Part model, mm, in its own coordinate system. A direction names the side the tool comes from. Give positions to 0.01 mm unless a question says otherwise; leave off trailing zeros. Write each loop counter-clockwise with the first axis right and the second up, starting at its lowest first coordinate (ties: lowest second). Pieces come first, ordered by that corner, then holes. Notation, with made-up numbers: M 84.5,29 L 110.5,29 A28 ccw 110.5,54 Z; hole C 1,72 d11. An arc over 180 degrees is marked long. Use CSV: the item, a comma, the result in double quotes. Start each with the question number.
Item 1: Cut at A-A (y = -48). List the corners of the cut face in (x, z), then the cut area to 3 significant figures.
Item 2: Cut at D-D (z = -6.75). List the corners of the cut face in (x, y), then the cut area to 3 significant figures.
Item 3: Which spindle directions (+Z, -Z, +X, -X, +Y, -Y) get a long thin tool onto all of the face, cutting with end or side? Do faces 5 (the flat face through (55.621, -33, -5)), 6 (the cylindrical face through (14.67, -52.925, -4.93)), 7 (the flat face through (15, 0, -5)). Say none if no direction does.
Item 4: Mould opens along X. For faces 1 (the flat face through (15, -67.016, -5)), 2 (the flat face through (15, -37.928, -5)), 3 (the cylindrical face through (37.22, -18.98, -4.93)), 4 (the flat face through (-17.7, 17.2, -4.9)) say: released by +X, released by -X, zero draft, split by the parting line, or undercut.
Item 5: Cut at B-B (x = 15). List the corners of the cut face in (y, z).
Item 6: Cut at C-C (x = 24). List the corners of the cut face in (y, z), then the cut area to 3 significant figures.
Item 7: Drill centre lines: line 1 (X direction, y = -12.5, z = -0.25); line 2 (X direction, y = -14, z = -7.5); line 3 (Y direction, x = 8.5, z = -3.5). Where is each one in solid material? Low to high. Write a range as [from, to].
Item 8: Pin check, flat tips, straight feed: pin 1 (12 mm diameter, centred on x = 0, y = -16.11, fed in from -Z); pin 2 (3 mm diameter, centred on x = 46, z = -3.5, fed in from +Y); pin 3 (1 mm diameter, centred on y = 13.5, z = -3, fed in from -X); pin 4 (3 mm diameter, centred on y = 13.5, z = -5.5, fed in from -X). Stop position of each tip, or through.
from build123d import *

# Parameters (mm, degrees)
SKETCH_1_R      = 7.5
EXTRUDE_1_DEPTH = 10


with BuildPart() as part:
    # 草圖1 → 填料-伸長1 (new body)
    with BuildSketch(Plane.XY):
        Polygon((-24.379405198, -67.016021468), (55.620594802, -67.016021468), (55.620594802, 2.983978532), (45.101238557, 32.144622287), (30, 0), (0, 0), (-11.19802439, 31.04197561), (-24.379405198, 2.983978532), align=None)
        with Locations((30.291786216, -16.110047004)):
            Circle(SKETCH_1_R, mode=Mode.SUBTRACT)
        with Locations((0, -16.110047004)):
            Circle(SKETCH_1_R, mode=Mode.SUBTRACT)
        with BuildLine():
            ThreePointArc((0, -37.928378378), (15, -52.928378378), (30, -37.928378378))
            Line((30, -37.928378378), (0, -37.928378378))
        make_face(mode=Mode.SUBTRACT)
    extrude(amount=-EXTRUDE_1_DEPTH)


solid = part.part
Worked answers:
1,outline,"M -24.38,-10 L 3.88,-10 L 3.88,0 L -24.38,0 Z; M 26.12,-10 L 55.62,-10 L 55.62,0 L 26.12,0 Z"
1,area,"578 mm^2"
2,outline,"M -24.38,-67.02 L 55.62,-67.02 L 55.62,2.98 L 45.1,32.14 L 30,0 L 0,0 L -11.2,31.04 L -24.38,2.98 Z; hole C 0,-16.11 d15; hole M 0,-37.93 A15 ccw 30,-37.93 Z; hole C 30.29,-16.11 d15"
2,area,"5,480 mm^2"
3,face 5,"+Z, -Z, +X, +Y, -Y"
3,face 6,"+Z, -Z"
3,face 7,"+Z, -Z, +Y"
4,face 1,"zero draft"
4,face 2,"undercut"
4,face 3,"undercut"
4,face 4,"released by -X"
5,outline,"M -67.02,-10 L -52.93,-10 L -52.93,0 L -67.02,0 Z; M -37.93,-10 L 0,-10 L 0,0 L -37.93,0 Z"
6,outline,"M -67.02,-10 L -49.93,-10 L -49.93,0 L -67.02,0 Z; M -37.93,-10 L -20.19,-10 L -20.19,0 L -37.93,0 Z; M -12.03,-10 L 0,-10 L 0,0 L -12.03,0 Z"
6,area,"469 mm^2"
7,line 1,"x = [-24.38, -6.57], [6.57, 23.72], [36.87, 55.62]"
7,line 2,"x = [-24.38, -7.2], [7.2, 23.09], [37.49, 55.62]"
7,line 3,"y = [-67.02, -51.45], [-37.93, 0]"
8,pin 1,"passes through"
8,pin 2,"stops at y = 32.14"
8,pin 3,"stops at x = -19.67"
8,pin 4,"stops at x = -20.14"
